from build123d import *

# Parameters (mm, degrees)
SKETCH1_W            = 96.4
SKETCH1_H            = 63
BOSS_EXTRUDE1_DEPTH  = 5.5
SKETCH1_5_W          = 93
SKETCH1_5_H          = 59.6
SKETCH1_5_W_2        = 86.9
SKETCH1_5_H_2        = 57
BOSS_EXTRUDE2_DEPTH  = 1.4
CHAMFER1_SIZE        = 1.5
SKETCH3_W            = 1.7
SKETCH3_H            = 13.2
BOSS_EXTRUDE4_DEPTH  = 1.7
SKETCH4_W            = 10
SKETCH4_H            = 1.7
SKETCH4_W_2          = 19.2
SKETCH4_W_3          = 13
BOSS_EXTRUDE5_DEPTH  = 1.6
SKETCH4_3_W          = 10
SKETCH4_3_H          = 1.7
SKETCH4_3_H_2        = 1.3
SKETCH4_3_W_2        = 19.2
SKETCH4_3_W_3        = 13
BOSS_EXTRUDE6_DEPTH  = 2
SKETCH3_5_W          = 3
SKETCH3_5_H          = 13.2
BOSS_EXTRUDE7_DEPTH  = 1
SKETCH5_W            = 1.7
SKETCH5_H            = 54.6
BOSS_EXTRUDE8_DEPTH  = 1.6
SKETCH5_3_W          = 1.3
SKETCH5_3_H          = 54.6
SKETCH5_3_W_2        = 1.7
BOSS_EXTRUDE9_DEPTH  = 2
SKETCH7_W            = 54.1
SKETCH7_H            = 8.9
CUT_EXTRUDE2_DEPTH   = 12
CHAMFER2_SIZE        = 1
SKETCH11_W           = 10
SKETCH11_H           = 2
SKETCH11_W_2         = 19.2
SKETCH11_W_3         = 13
BOSS_EXTRUDE10_DEPTH = 2
SKETCH13_W           = 10
SKETCH13_H           = 2
SKETCH13_W_2         = 19.2
SKETCH13_W_3         = 13
BOSS_EXTRUDE12_DEPTH = 0.9
SKETCH14_W           = 54.1
SKETCH14_H           = 3
BOSS_EXTRUDE13_DEPTH = 2.9
SKETCH15_W           = 2
SKETCH15_H           = 54.6
BOSS_EXTRUDE14_DEPTH = 4.5
SKETCH16_W           = 3.5
SKETCH16_H           = 54.6
BOSS_EXTRUDE15_DEPTH = 0.8
SKETCH18_R           = 3.5
CUT_EXTRUDE4_DEPTH   = 12
CUT_EXTRUDE5_DEPTH   = 4.3


with BuildPart() as part:
    # Sketch1 → Boss-Extrude1 (new body)
    with BuildSketch(Plane.XY):
        with Locations((10.058192988, -1.431154761)):
            Rectangle(SKETCH1_W, SKETCH1_H)
    extrude(amount=BOSS_EXTRUDE1_DEPTH)

    # Sketch1_5 → Boss-Extrude2 (add)
    # profile 1 of 2: a face of its own
    with BuildSketch(Plane.XY):
        with Locations((10.058192988, -1.431154761)):
            Rectangle(SKETCH1_5_W, SKETCH1_5_H)
        with Locations((11.808192988, -1.431154761)):
            Rectangle(SKETCH1_5_W_2, SKETCH1_5_H_2, mode=Mode.SUBTRACT)
    # profile 2 of 2: a face of its own
    with BuildSketch(Plane.XY):
        with Locations((11.808192988, -1.431154761)):
            Rectangle(SKETCH1_5_W_2, SKETCH1_5_H_2)
    extrude(amount=-BOSS_EXTRUDE2_DEPTH)

    # Chamfer1
    chamfer1_edges = [part.edges().sort_by_distance(p)[0] for p in [
        (-38.141807012, 30.068845239, 2.75),
        (58.258192988, 30.068845239, 2.75),
        (58.258192988, -32.931154761, 2.75),
        (-38.141807012, -32.931154761, 2.75),
    ]]
    chamfer(chamfer1_edges, length=CHAMFER1_SIZE)

    # Sketch3 → Boss-Extrude4 (add)
    with BuildSketch(Plane(origin=(0, 0, -1.4), x_dir=(-1, 0, 0), z_dir=(0, 0, -1))):
        with Locations((37.291807012, -1.631154761)):
            Rectangle(SKETCH3_W, SKETCH3_H)
    extrude(amount=-BOSS_EXTRUDE4_DEPTH)

    # Sketch4 → Boss-Extrude5 (add)
    with BuildSketch(Plane(origin=(0, 0, -1.4), x_dir=(-1, 0, 0), z_dir=(0, 0, -1))):
        with Locations((-22.068192988, 29.218845239)):
            Rectangle(SKETCH4_W, SKETCH4_H)
        with Locations((-0.358192988, 29.218845239)):
            Rectangle(SKETCH4_W_2, SKETCH4_H)
        with Locations((20.741807012, 29.218845239)):
            Rectangle(SKETCH4_W_3, SKETCH4_H)
    extrude(amount=-BOSS_EXTRUDE5_DEPTH)

    # Sketch4_3 → Boss-Extrude6 (add)
    with BuildSketch(Plane(origin=(0, 0, -1.4), x_dir=(-1, 0, 0), z_dir=(0, 0, -1))):
        with Locations((-22.068192988, 29.218845239)):
            Rectangle(SKETCH4_3_W, SKETCH4_3_H)
        with Locations((-22.068192988, 27.718845239)):
            Rectangle(SKETCH4_3_W, SKETCH4_3_H_2)
        with Locations((-0.358192988, 27.718845239)):
            Rectangle(SKETCH4_3_W_2, SKETCH4_3_H_2)
        with Locations((-0.358192988, 29.218845239)):
            Rectangle(SKETCH4_3_W_2, SKETCH4_3_H)
        with Locations((20.741807012, 27.718845239)):
            Rectangle(SKETCH4_3_W_3, SKETCH4_3_H_2)
        with Locations((20.741807012, 29.218845239)):
            Rectangle(SKETCH4_3_W_3, SKETCH4_3_H)
    extrude(amount=BOSS_EXTRUDE6_DEPTH)

    # Sketch3_5 → Boss-Extrude7 (add)
    with BuildSketch(Plane(origin=(0, 0, -1.4), x_dir=(-1, 0, 0), z_dir=(0, 0, -1))):
        with Locations((36.641807012, -1.631154761)):
            Rectangle(SKETCH3_5_W, SKETCH3_5_H)
    extrude(amount=BOSS_EXTRUDE7_DEPTH)

    # Sketch5 → Boss-Extrude8 (add)
    with BuildSketch(Plane(origin=(0, 0, -1.4), x_dir=(-1, 0, 0), z_dir=(0, 0, -1))):
        with Locations((-57.408192988, -2.231154761)):
            Rectangle(SKETCH5_W, SKETCH5_H)
    extrude(amount=-BOSS_EXTRUDE8_DEPTH)

    # Sketch5_3 → Boss-Extrude9 (add)
    with BuildSketch(Plane(origin=(0, 0, -1.4), x_dir=(-1, 0, 0), z_dir=(0, 0, -1))):
        with Locations((-55.908192988, -2.231154761)):
            Rectangle(SKETCH5_3_W, SKETCH5_3_H)
        with Locations((-57.408192988, -2.231154761)):
            Rectangle(SKETCH5_3_W_2, SKETCH5_3_H)
    extrude(amount=BOSS_EXTRUDE9_DEPTH)

    # Sketch7 → Cut-Extrude2 (cut)
    with BuildSketch(Plane.XY.offset(5.5)):
        with Locations((1.008192988, -25.481154761)):
            Rectangle(SKETCH7_W, SKETCH7_H)
    extrude(amount=-CUT_EXTRUDE2_DEPTH, mode=Mode.SUBTRACT)

    # Chamfer2
    chamfer2_edges = [part.edges().sort_by_distance(p)[0] for p in [
        (28.058192988, -29.931154761, 2.05),
        (-26.041807012, -29.931154761, 2.05),
        (-26.041807012, -21.031154761, 2.05),
        (28.058192988, -21.031154761, 2.05),
    ]]
    chamfer(chamfer2_edges, length=CHAMFER2_SIZE)

    # Sketch11 → Boss-Extrude10 (add)
    with BuildSketch(Plane.XZ.offset(-27.068845239)):
        with Locations((22.068192988, -2.4)):
            Rectangle(SKETCH11_W, SKETCH11_H)
        with Locations((0.358192988, -2.4)):
            Rectangle(SKETCH11_W_2, SKETCH11_H)
        with Locations((-20.741807012, -2.4)):
            Rectangle(SKETCH11_W_3, SKETCH11_H)
    extrude(amount=BOSS_EXTRUDE10_DEPTH)

    # Sketch13 → Boss-Extrude12 (add)
    with BuildSketch(Plane(origin=(0, 0, -3.4), x_dir=(-1, 0, 0), z_dir=(0, 0, -1))):
        with Locations((-22.068192988, 26.068845239)):
            Rectangle(SKETCH13_W, SKETCH13_H)
        with Locations((-0.358192988, 26.068845239)):
            Rectangle(SKETCH13_W_2, SKETCH13_H)
        with Locations((20.741807012, 26.068845239)):
            Rectangle(SKETCH13_W_3, SKETCH13_H)
    extrude(amount=BOSS_EXTRUDE12_DEPTH)

    # Sketch14 → Boss-Extrude13 (add)
    with BuildSketch(Plane(origin=(0, 0, -1.4), x_dir=(-1, 0, 0), z_dir=(0, 0, -1))):
        with Locations((-1.008192988, -19.531154761)):
            Rectangle(SKETCH14_W, SKETCH14_H)
    extrude(amount=BOSS_EXTRUDE13_DEPTH)

    # Sketch15 → Boss-Extrude14 (add)
    with BuildSketch(Plane.ZY.offset(-55.258192988)):
        with Locations((-2.4, -2.231154761)):
            Rectangle(SKETCH15_W, SKETCH15_H)
    extrude(amount=BOSS_EXTRUDE14_DEPTH)

    # Sketch16 → Boss-Extrude15 (add)
    with BuildSketch(Plane(origin=(0, 0, -3.4), x_dir=(-1, 0, 0), z_dir=(0, 0, -1))):
        with Locations((-52.508192988, -2.231154761)):
            Rectangle(SKETCH16_W, SKETCH16_H)
    extrude(amount=BOSS_EXTRUDE15_DEPTH)

    # Sketch18 → Cut-Extrude4 (cut)
    with BuildSketch(Plane(origin=(0, 0, -1.4), x_dir=(-1, 0, 0), z_dir=(0, 0, -1))):
        with Locations((-41.058192988, -1.431154761)):
            Circle(SKETCH18_R)
        with Locations((-25.558192988, -1.431154761)):
            Circle(SKETCH18_R)
        with Locations((-10.058192988, -1.431154761)):
            Circle(SKETCH18_R)
        with Locations((5.441807012, -1.431154761)):
            Circle(SKETCH18_R)
        with Locations((20.941807012, -1.431154761)):
            Circle(SKETCH18_R)
    extrude(amount=-CUT_EXTRUDE4_DEPTH, mode=Mode.SUBTRACT)

    # Sketch18_3 → Cut-Extrude5 (cut)
    with BuildSketch(Plane(origin=(0, 0, -1.4), x_dir=(-1, 0, 0), z_dir=(0, 0, -1))):
        Polygon((-41.058192988, -8.070682857), (-35.308192988, -4.750918809), (-35.308192988, 1.888609286), (-41.058192988, 5.319984429), (-46.808192988, 1.888609286), (-46.808192988, -4.750918809), align=None)
        Polygon((-25.558192988, 5.208373334), (-31.308192988, 1.888609286), (-31.308192988, -4.750918809), (-25.558192988, -8.070682857), (-19.808192988, -4.750918809), (-19.808192988, 1.888609286), align=None)
        Polygon((-10.058192988, 5.208373334), (-15.808192988, 1.888609286), (-15.808192988, -4.750918809), (-10.058192988, -8.070682857), (-4.308192988, -4.750918809), (-4.308192988, 1.888609286), align=None)
        Polygon((5.441807012, 5.208373334), (-0.308192988, 1.888609286), (-0.308192988, -4.750918809), (5.441807012, -8.070682857), (11.191807012, -4.750918809), (11.191807012, 1.888609286), align=None)
        Polygon((20.941807012, 5.208373334), (15.191807012, 1.888609286), (15.191807012, -4.750918809), (20.941807012, -8.070682857), (26.691807012, -4.750918809), (26.691807012, 1.888609286), align=None)
    extrude(amount=-CUT_EXTRUDE5_DEPTH, mode=Mode.SUBTRACT)


solid = part.part
Design review of the part built by this model. Coordinates are the model's own, in mm. A direction names the side the tool comes from. Round coordinates to 2 decimals unless told otherwise and drop trailing zeros. Write each loop counter-clockwise with the first axis right and the second up, starting at its lowest first coordinate (ties: lowest second). Pieces come first, ordered by that corner, then holes. Notation, with made-up numbers: (70.5, 12.25) - (90.5, 12.25) arc R16 cw to (90.5, 36.25) - close; hole circle Ø7 at (63, 45.25). An arc over 180 degrees is marked (long way). Return JSON: item names as keys, results as strings. Group by question number.
Item 1: We need section B-B on x = 24.5. Write out the cut boundary in (y, z).
Item 2: Machinability: for faces 4 (the face through (38.14, 3.58, 0.72)), 5 (the face through (22, 25.069, -3)), 6 (the face through (-21, 26, -4.3)), which of the approach directions +Z, -Z, +X, -X, +Y, -Y give a long, thin tool a straight path to every point of the face, cutting with its end or side? Answer none if there is none.
Item 3: We need section A-A on y = 17. Write out the cut boundary in (x, z).
Item 4: We need section C-C on z = 1.75. Give the number of separate pieces and of enclosed holes in the cut face, and give its area (3 significant figures).
Item 5: For probe 1 along Y at (x, z) = (16.5, 2.5); probe 2 along Y at (x, z) = (5.5, -1.25); probe 3 along X at (y, z) = (-3, 2), list the stretches that pass through material, from the lowest coordinate up. Write a range as [from, to].
Item 6: The part is to be moulded in two halves that separate along X. For faces 1 (the face through (28.058, -26, 2)), 2 (the face through (58.258, -2, 1)), 3 (the face through (1, -20, -4.3)), say which applies: pulls with the +X half, pulls with the -X half, needs draft (parallel to the pull), parting line crosses it, or undercut.
Item 7: Insertion check: P1, Ø1.5, axis at x = 40.5, y = 27.5, coming from the -Z side; P2, Ø2.5, axis at y = -19, z = -3, coming from the -X side; P3, Ø1.3, axis at x = 53.5, z = -2, coming from the -Y side. Each pin has a flat end and moves straight along its axis. Give the tip position at first contact, or say it passes through.
Model answer:
{
 "1": {"outline": "(-32.93, 0) - (-31.23, 0) - (-31.23, -1.4) - (-29.93, -1.4) - (-29.93, 5.5) - (-32.93, 5.5) - close; (-21.03, -4.3) - (-18.03, -4.3) - (-18.03, -1.4) - (-7.46, -1.4) - (-7.46, 2.9) - (-4.77, 2.9) - (-4.77, 5.5) - (-21.03, 5.5) - close; (1.91, 2.9) - (4.6, 2.9) - (4.6, -1.4) - (25.07, -1.4) - (25.07, -4.3) - (27.07, -4.3) - (27.07, -3.4) - (30.07, -3.4) - (30.07, 5.5) - (1.91, 5.5) - close"},
 "2": {"face 4": "-Z", "face 5": "-Z, -X", "face 6": "-Z, +X, -X, +Y, -Y"},
 "3": {"outline": "(-38.14, 0) - (-36.44, 0) - (-36.44, -1.4) - (50.76, -1.4) - (50.76, -4.2) - (54.26, -4.2) - (54.26, -3.4) - (58.26, -3.4) - (58.26, 5.5) - (-38.14, 5.5) - close"},
 "4": {"separate pieces": "1", "enclosed holes": "6", "area": "5,020 mm²"},
 "5": {"probe 1": "y = [-32.93, -29.93], [-21.03, 30.07]", "probe 2": "y = [-31.23, -29.93], [-21.03, -5.44], [2.58, 30.07]", "probe 3": "x = [-38.14, -26.69], [-15.19, -11.19], [0.31, 4.31], [15.81, 19.81], [31.31, 35.31], [46.81, 58.26]"},
 "6": {"face 1": "undercut", "face 2": "pulls with the +X half", "face 3": "needs draft"},
 "7": {"P1": "stops at z = -1.4", "P2": "stops at x = -26.04", "P3": "stops at y = -31.23"}
}
